Can you work these out from the drawing? Everything is in mm from the part's minimum corner. A direction names the side the tool comes from. Round coordinates to 2 decimals unless told otherwise and drop trailing zeros. Write each loop counter-clockwise with the first axis right and the second up, starting at its lowest first coordinate (ties: lowest second). Pieces come first, ordered by that corner, then holes. Notation, with made-up numbers: (57, -8.5) - (78, -8.5) arc R16 cw to (78, 14.5) - close; hole circle Ø4 at (14.25, 10). An arc over 180 degrees is marked (long way). One line per item, written item: value. Start each with the question number.
Item 1: If I drill on line 1 (Y direction, x = 5, z = 1.45); line 2 (Z direction, x = 1.5, y = 2); line 3 (Y direction, x = 6, z = 0.3), over which ranges is the centre line in solid material (lowest first)?
Item 2: Imagine slicing it at C-C, the plane z = 1.9. Please give me the cut outline in (x, y), then the cut area to 3 significant figures.
Item 3: Imagine slicing it at D-D, the plane x = 1. Please give me the cut outline in (y, z), then the cut area to 3 significant figures.
Item 4: For P1, Ø1.5, axis at y = 1.5, z = 0.5, coming from the +X side, with a flat end and sliding along its axis, tell me the tip position at first contact or that it passes through.
Item 5: Thinking about a two-plate mould opening in Z: for the marked faces 1, 2 and 3, which applies, released by +Z, released by -Z, zero draft, split by the parting line, or undercut?
Item 6: Imagine slicing it at A-A, the plane y = 5. Please give me the cut outline in (x, z).
Item 7: For the marked faces 4 and 5, which set-ups out of +Z, -Z, +X, -X, +Y, -Y let a thin tool reach every point of the face, with its end or its side?
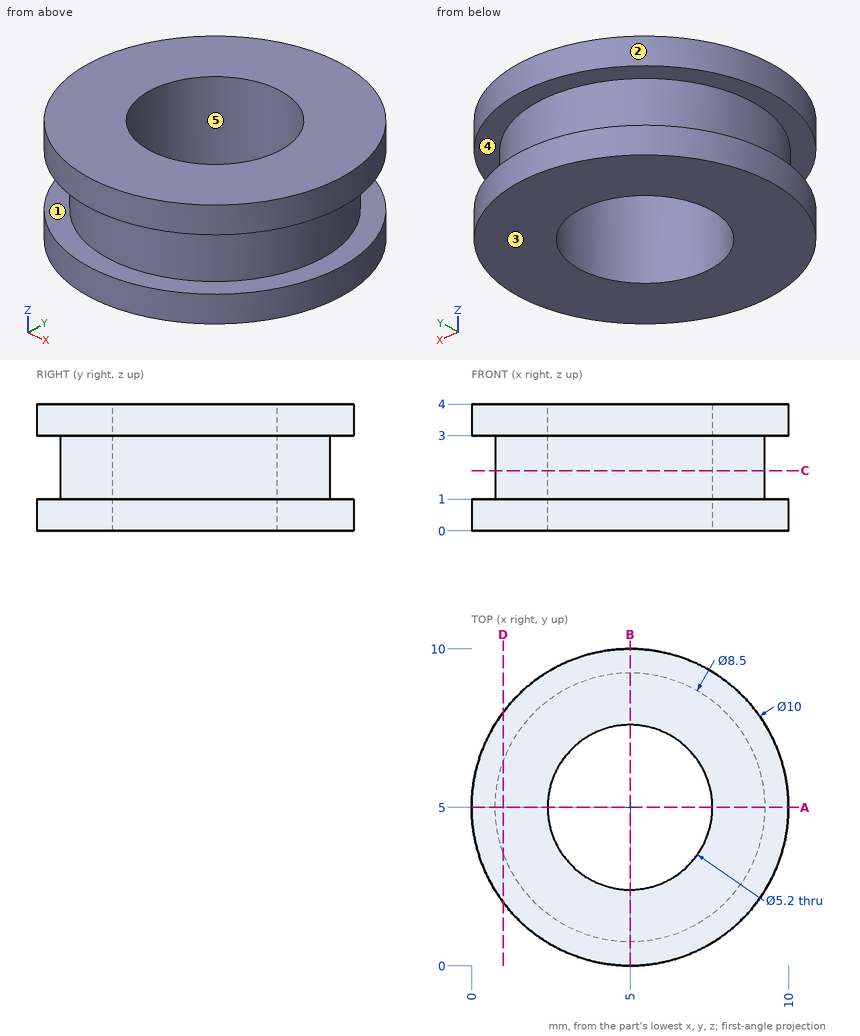
Values follow:
1. line 1: y = 0.75 to 2.4, 7.6 to 9.25
1. line 2: z = 0 to 1, 3 to 4
1. line 3: y = 0.1 to 2.6, 7.4 to 9.9
2. outline: circle Ø8.5 at (5, 5); hole circle Ø5.2 at (5, 5)
2. area: 35.5 mm^2
3. outline: (2, 0) - (8, 0) - (8, 1) - (6.44, 1) - (6.44, 3) - (8, 3) - (8, 4) - (2, 4) - (2, 3) - (3.56, 3) - (3.56, 1) - (2, 1) - close
3. area: 17.7 mm^2
4. P1: stops at x = 9.18
5. face 1: undercut
5. face 2: zero draft
5. face 3: released by -Z
6. outline: (0, 0) - (2.4, 0) - (2.4, 4) - (0, 4) - (0, 3) - (0.75, 3) - (0.75, 1) - (0, 1) - close; (7.6, 0) - (10, 0) - (10, 1) - (9.25, 1) - (9.25, 3) - (10, 3) - (10, 4) - (7.6, 4) - close
7. face 4: none
7. face 5: +Z, -Z
